Design review of the part built by this model. Coordinates are the model's own, in mm. Face numbers are marked on the shaded views. A direction names the side the tool comes from. Give positions to 0.01 mm unless a question says otherwise; leave off trailing zeros. Loops run counter-clockwise (first coordinate to the right, second up) from the corner with the lowest first, then second, coordinate; pieces in that order, holes last. Notation, with made-up numbers: (17, -26) -> (74, -26) arc R23 cw to (74, -13) -> close; hole circle Ø2 at (-25.5, 69). An arc over 180 degrees is marked (long way). Answer in a Markdown table with one row per item. Add a question column.
(1) For pin 1 (5 mm diameter, centred on x = -1, y = -11.5, fed in from -Z); pin 2 (2 mm diameter, centred on x = 8.5, y = -22, fed in from +Z), all flat-tipped, find the tip position at first contact; note any pin that passes through.
(2) For the marked faces 4 and 5, list the 3-axis set-ups (+Z, -Z, +X, -X, +Y, -Y) from which the entire face can be reached by the end or side of a thin tool; tool diameter is ignored.
(3) Draft analysis for pull direction X (two halves, no side actions). For the marked faces 1, 2 and 3, state which applies: +X half, -X half, draft (parallel to the pull), parting line (faces both ways), or undercut.
(4) For line 1 (Y direction, x = -8.5, z = 2.6); line 2 (X direction, y = -3, z = 3.45); line 3 (X direction, y = -2, z = -0.25), list the stretches that pass through material, from the lowest coordinate up.
(5) Consider section C-C on x = -3.5. Write out the cut boundary in (y, z), then the cut area to 3 significant figures.
(6) Consider section A-A on z = 2.5. Write out the cut boundary in (x, y), then the cut area to 3 significant figures.
(7) Consider section B-B on y = -8.25. Write out the cut boundary in (x, z).
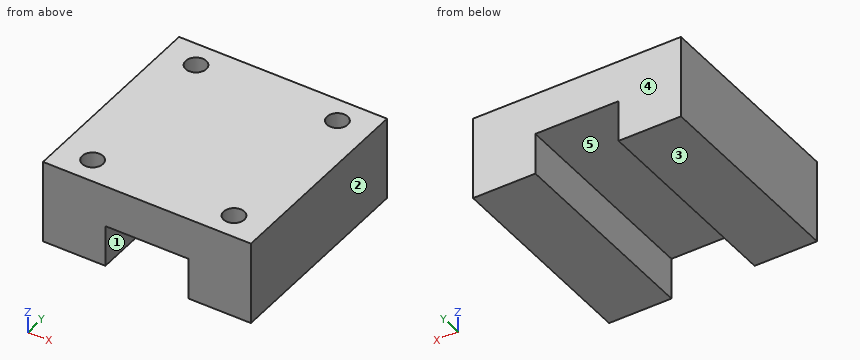
from build123d import *

# Parameters (mm, degrees)
F1_DEPTH = 25
F3_D     = 2.5
F3_DEPTH = 5
F3_TIP   = 0.7510757738


with BuildPart() as f1:
    # F0 (on Front) → F1 (new body)
    with BuildSketch(Plane.XZ):
        Polygon((-5, 0), (0, 0), (5, 0), (5, -5), (12.5, -5), (12.5, 5), (0, 5), (-12.5, 5), (-12.5, -5), (-5, -5), align=None)
    extrude(amount=F1_DEPTH)

    # F3
    with Locations(Plane.XY.offset(5)):
        with Locations((-8.5, -3), (8.5, -3), (-8.5, -22), (8.5, -22)):
            Hole(F3_D / 2, depth=F3_DEPTH)
            with Locations((0, 0, -(F3_DEPTH + F3_TIP / 2))):  # 118° drill point
                Cone(0, F3_D / 2, F3_TIP, mode=Mode.SUBTRACT)


solid = f1.part
Values follow:
| question | item | result |
|---|---|---|
| 1 | pin 1 | z = 0 |
| 1 | pin 2 | z = -0.15 |
| 2 | face 4 | +Z, -Z, +X, -X, +Y |
| 2 | face 5 | -Z, +Y, -Y |
| 3 | face 1 | undercut |
| 3 | face 2 | +X half |
| 3 | face 3 | draft |
| 4 | line 1 | -25 to -23.25, -20.75 to -4.25, -1.75 to 0 |
| 4 | line 2 | -12.5 to -9.75, -7.25 to 7.25, 9.75 to 12.5 |
| 4 | line 3 | -12.5 to -5, 5 to 12.5 |
| 5 | outline | (-25, 0) -> (0, 0) -> (0, 5) -> (-25, 5) -> close |
| 5 | area | 125 mm2 |
| 6 | outline | (-12.5, -25) -> (12.5, -25) -> (12.5, 0) -> (-12.5, 0) -> close; hole circle Ø2.5 at (-8.5, -22); hole circle Ø2.5 at (-8.5, -3); hole circle Ø2.5 at (8.5, -22); hole circle Ø2.5 at (8.5, -3) |
| 6 | area | 605 mm2 |
| 7 | outline | (-12.5, -5) -> (-5, -5) -> (-5, 0) -> (5, 0) -> (5, -5) -> (12.5, -5) -> (12.5, 5) -> (-12.5, 5) -> close |
